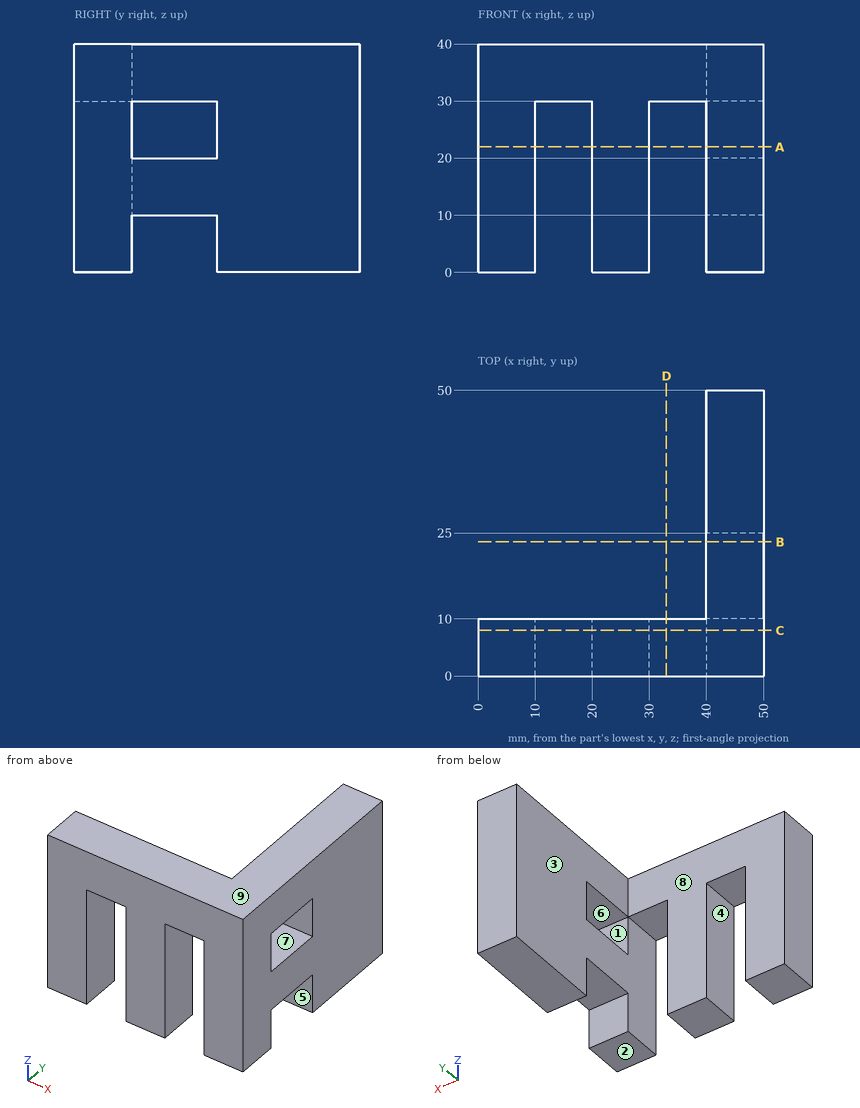
Input: dimensioned drawing with shaded views. Units: mm. Origin: part minimum x, y, z. A direction names the side the tool comes from. Give positions to 0.01 mm unless a question says otherwise; leave off trailing zeros. Write each loop counter-clockwise with the first axis right and the second up, starting at its lowest first coordinate (ties: lowest second). Pieces come first, ordered by that corner, then holes.
Q1. Section C-C, the plane y = 8. Output: boundary loops of the cut face in (x, z).
Q2. Section B-B, the plane y = 23.5. Output: boundary loops of the cut face in (x, z).
Q3. Material intervals for probe 1 along X at (y, z) = (6, 13); probe 2 along Y at (x, z) = (48.5, 21.5); probe 3 along X at (y, z) = (37.5, 6), sorted ascending.
Q4. Section A-A, the plane z = 22. Output: boundary loops of the cut face in (x, y).
Q5. Set-up query: the marked faces 1, 2, 3, 4 and 5. Return all of +Z, -Z, +X, -X, +Y, -Y with unobstructed straight access to the full face (end or side cutting, diameter ignored); none if empty.
Q6. First-contact query: P1, Ø11, axis at x = 34.5, y = 4.5, coming from the -Z side; P2, Ø5, axis at x = 47, y = 21, coming from the -Z side; P3, Ø10, axis at x = 15.5, z = 25, coming from the +Y side; P4, Ø3, axis at x = 15, y = 5, coming from the -Z side. Flat tips, straight axial feed; report the tip coordinate or a pass-through.
Q7. Section D-D, the plane x = 33. Output: boundary loops of the cut face in (y, z).
Q8. Pull-direction query (Y, two-part tool) for the marked faces 6, 7, 8 and 9; classes: pulls with the +Y half, pulls with the -Y half, needs draft (parallel to the pull), parting line crosses it, or undercut.
Filled in:
1. outline: (0, 0) - (10, 0) - (10, 30) - (20, 30) - (20, 0) - (30, 0) - (30, 30) - (40, 30) - (40, 0) - (50, 0) - (50, 40) - (0, 40) - close
2. outline: (40, 10) - (50, 10) - (50, 20) - (40, 20) - close; (40, 30) - (50, 30) - (50, 40) - (40, 40) - close
3. probe 1: x = 0 to 10, 20 to 30, 40 to 50
3. probe 2: y = 0 to 10, 25 to 50
3. probe 3: x = 40 to 50
4. outline: (0, 0) - (10, 0) - (10, 10) - (0, 10) - close; (20, 0) - (30, 0) - (30, 10) - (20, 10) - close; (40, 0) - (50, 0) - (50, 10) - (40, 10) - close; (40, 25) - (50, 25) - (50, 50) - (40, 50) - close
5. face 1: +X, -X
5. face 2: -Z, +X, -X, +Y, -Y
5. face 3: -Z, +Y
5. face 4: -Z, +Y, -Y
5. face 5: -Z, +X, -X
6. P1: stops at z = 0
6. P2: stops at z = 10
6. P3: stops at y = 10
6. P4: stops at z = 30
7. outline: (0, 30) - (10, 30) - (10, 40) - (0, 40) - close
8. face 6: undercut
8. face 7: undercut
8. face 8: pulls with the +Y half
8. face 9: needs draft
